Input: part model. Units: mm. Frame: model coordinates. A direction names the side the tool comes from. Round coordinates to 2 decimals unless told otherwise and drop trailing zeros. Loops run counter-clockwise (first coordinate to the right, second up) from the corner with the lowest first, then second, coordinate; pieces in that order, holes last. Notation, with made-up numbers: (1.5, 80.25) -> (6.5, 80.25) arc R19 ccw to (6.5, 107.25) -> close; hole circle Ø5 at (68.25, 56.25). An arc over 180 degrees is marked (long way). Answer as a JSON object with one key per item and string values.
```python
from build123d import *

# Parameters (mm, degrees)
F0_W     = 4.7625
F0_H     = 35.56
F2_R     = 2.54
F3_DEPTH = 7.62


with BuildPart() as f1:
    # F0 (on Front) → F1 (revolve)
    with BuildSketch(Plane.XZ):
        Polygon((0, 25.4), (0, 15.24), (6.35, 15.24), align=None)
        Polygon((0, 10.16), (4.7625, 10.16), (6.35, 10.16), (6.35, 15.24), (0, 15.24), align=None)
        with Locations((2.38125, -7.62)):
            Rectangle(F0_W, F0_H)
    revolve(axis=Axis((0, 0, 0), (0, 0, -1)))

    # F2 (on Right) → F3 (cut)
    with BuildSketch(Plane.YZ):
        with Locations((0, -17.78)):
            Circle(F2_R)
    extrude(amount=-F3_DEPTH, mode=Mode.SUBTRACT)


solid = f1.part
```
1) Ray query, probe 1 along Z at (x, y) = (-1.85, 0); probe 2 along Z at (x, y) = (-1.5, 0); probe 3 along Y at (x, z) = (-3.3, -17.78). Return the intervals inside material, ascending.
Output:
{"probe 1": "z = -25.4 to -20.32, -15.24 to 22.44", "probe 2": "z = -25.4 to -20.32, -15.24 to 23", "probe 3": "y = -3.43 to -2.54, 2.54 to 3.43"}
2) Contact query for flat-ended pins moving along their axis: P1, Ø2, axis at y = -3, z = -12, coming from the +X side; P2, Ø5, axis at x = -2.5, y = 1, coming from the +Z side; P3, Ø6, axis at y = -3.5, z = 11, coming from the +X side. Output: stop coordinate, or through.
Output:
{"P1": "stops at x = 4.32", "P2": "stops at z = 25.09", "P3": "stops at x = 6.33"}
3) Section A-A, the plane z = 2.5. Output: boundary loops of the cut face in (x, y) (1 decimal), plus the area to 3 significant figures.
Output:
{"outline": "circle Ø9.5 at (0, 0)", "area": "71.3 mm^2"}
4) Reachability of faces 1 (the face through (0, 0, -18)), 2 (the face through (4.543, -1.431, -7.371)), 3 (the face through (0, 0, -25.4)) from +Z, -Z, +X, -X, +Y, -Y: full face, straight path, thin tool, end or side. Return the list, or none.
Output:
{"face 1": "-X", "face 2": "-Z", "face 3": "-Z, +X, -X, +Y, -Y"}
5) Draft query along Z for faces 4 (the face through (-1, -5, 10.16)), 5 (the face through (2.24, 0.93, 21.52)), 6 (the face through (-2.351, 2.423, -17.017)). Return one class per face: +Z half, -Z half, draft (parallel to the pull), parting line (faces both ways), or undercut.
Output:
{"face 4": "-Z half", "face 5": "+Z half", "face 6": "undercut"}
